Autodesk Inventor part; units mm, degrees
ref_plane "YZ Plane" through (0, 0, 0) normal (1, 0, 0) x (0, 1, 0)
ref_plane "XZ Plane" through (0, 0, 0) normal (0, 1, 0) x (-1, 0, 0)
ref_plane "XY Plane" through (0, 0, 0) normal (0, 0, 1) x (1, 0, 0)
sketch "Sketch1" plane through (0, 0, 0) normal (0, 0, 1) x (1, 0, 0)
  line L0 (0, 0) -> (25.4, 0)
  line L1 (25.4, 0) -> (25.4, -50.8)
  line L2 (25.4, -50.8) -> (0, -50.8)
  line L3 (0, -50.8) -> (0, 0)
  line L4 (22.225, -3.175) -> (3.175, -3.175)
  line L5 (3.175, -3.175) -> (3.175, -47.625)
  line L6 (3.175, -47.625) -> (22.225, -47.625)
  line L7 (22.225, -47.625) -> (22.225, -3.175)
  dimension "d0" = 25.4
  dimension "d1" = 50.8
  dimension "d2" = 3.175
  dimension "d3" = 3.175
  dimension "d4" = 3.175
  dimension "d5" = 3.175
extrude "Extrusion1" add sketch "Sketch1" along normal blind 76.2
sketch "Sketch2" plane through (0, -50.8, 0) normal (-1, 0, 0) x (0, 0, 1)
  circle A0 centre (57.15, 25.4) radius 14.2875
  line L0 (76.2, 50.8) -> (76.2, 0)
  line L1 (0, 50.8) -> (76.2, 50.8)
  dimension "d8" = 28.575
  dimension "d9" = 19.05
  dimension "d10" = 25.4
extrude "Extrusion2" cut sketch "Sketch2" against normal through all
sketch "Sketch3" plane through (0, -50.8, 0) normal (-1, 0, 0) x (0, 0, 1)
  line L0 (76.2, 47.625) -> (76.2, 3.175)
  line L1 (76.2, 31.75) -> (57.15, 50.8)
  line L2 (0, 50.8) -> (76.2, 50.8)
  line L3 (76.2, 0) -> (76.2, 50.8)
  line L4 (57.15, 50.8) -> (76.2, 50.8)
  line L5 (76.2, 50.8) -> (76.2, 31.75)
  dimension "d13" = 135
  dimension "d14" = 19.05
extrude "Extrusion3" cut sketch "Sketch3" against normal through all
sketch "Sketch4" plane through (0, -50.8, 0) normal (-1, 0, 0) x (0, 0, 1)
  circle A0 centre (12.7, 12.7) radius 3.3734
  circle A1 centre (12.7, 38.1) radius 3.3734
  line L0 (0, 50.8) -> (57.15, 50.8)
  line L1 (0, 0) -> (0, 50.8)
  dimension "d17" = 6.7469
  dimension "d18" = 12.7
  dimension "d19" = 38.1
  dimension "d20" = 12.7
  dimension "d21" = 12.7
extrude "Extrusion4" cut sketch "Sketch4" against normal blind 25.4
properties part number "flywheelsupport2" material "Aluminum 6061"
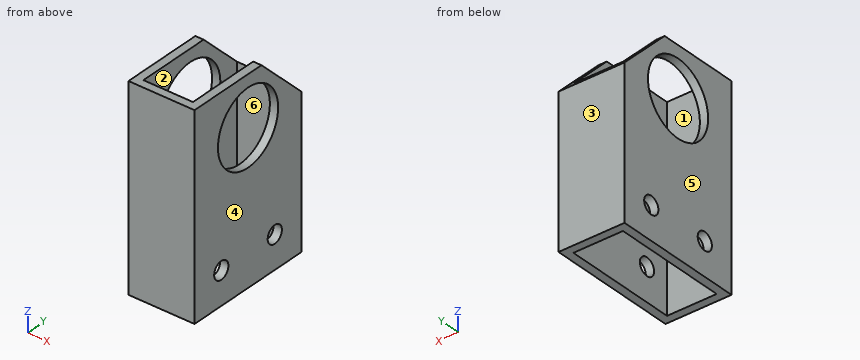
Geometry check sheet. Reference: the model listing, model coordinates, mm. Face numbers are marked on the shaded views. A direction names the side the tool comes from. Give positions to 0.01 mm unless a question says otherwise; leave off trailing zeros. Loops run counter-clockwise (first coordinate to the right, second up) from the corner with the lowest first, then second, coordinate; pieces in that order, holes last. Notation, with made-up numbers: (72.5, -13) - (115.5, -13) arc R31 ccw to (115.5, 20) - close; hole circle Ø5 at (42, 10.25). An arc over 180 degrees is marked (long way). Use CSV: the item, a comma, the result in double quotes. Start each with the question number.
Q1. Go/stop test with a flat-tipped pin: pin 1 Ø6 at (x, y) = (21, -13) entering from +Z. Record where the tip stops, or that it passes through.
Q2. Access from +Z, -Z, +X, -X, +Y, -Y to the whole of each face (thin tool, end or side, straight path). Record for the marked faces 5 and 6.
Q3. Section check C-C, the plane z = 24.5. Record the cut outline in (x, y) (3 decimals), and give its area (3 significant figures).
Q4. Section check D-D, the plane z = 12.7. Record the cut outline in (x, y) (3 decimals), and give its area (3 significant figures).
Q5. Section check A-A, the plane y = -44. Record the cut outline in (x, z) (3 decimals), and give its area (3 significant figures).
Q6. Release check for a two-part mould opening along X. For the marked faces 1, 2, 3 and 4 record: +X half, -X half, draft (parallel to the pull), parting line (faces both ways), or undercut.
Q7. Scan lines: probe 1 along Y at (x, z) = (1.4, 12.7); probe 2 along X at (y, z) = (-44, 25) (3 decimals); probe 3 along Y at (x, z) = (3.5, 24.5) (3 decimals). Record each from-to range of solid material in increasing order. Write a range as from..to.
Q8. Section check B-B, the plane x = 13.75. Record the cut outline in (y, z) (3 decimals).
Findings below:
1,pin 1,"stops at z = 72.89"
2,face 5,"+Z, -Z, -X, +Y, -Y"
2,face 6,"+Z, -Z"
3,outline,"(0, -50.8) - (25.4, -50.8) - (25.4, 0) - (0, 0) - close; hole (3.175, -47.625) - (22.225, -47.625) - (22.225, -3.175) - (3.175, -3.175) - close"
3,area,"444 mm^2"
4,outline,"(0, -50.8) - (25.4, -50.8) - (25.4, -41.473) - (22.225, -41.473) - (22.225, -47.625) - (3.175, -47.625) - (3.175, -41.473) - (0, -41.473) - close; (0, -34.727) - (3.175, -34.727) - (3.175, -16.073) - (0, -16.073) - close; (0, -9.327) - (3.175, -9.327) - (3.175, -3.175) - (22.225, -3.175) - (22.225, -9.327) - (25.4, -9.327) - (25.4, 0) - (0, 0) - close; (22.225, -34.727) - (25.4, -34.727) - (25.4, -16.073) - (22.225, -16.073) - close"
4,area,"358 mm^2"
5,outline,"(0, 0) - (3.175, 0) - (3.175, 76.2) - (0, 76.2) - close; (22.225, 0) - (25.4, 0) - (25.4, 76.2) - (22.225, 76.2) - close"
5,area,"484 mm^2"
6,face 1,"undercut"
6,face 2,"undercut"
6,face 3,"draft"
6,face 4,"+X half"
7,probe 1,"y = -50.8..-41.47, -34.73..-16.07, -9.33..0"
7,probe 2,"x = 0..3.175, 22.225..25.4"
7,probe 3,"y = -50.8..-47.625, -3.175..0"
8,outline,"(-50.8, 0) - (-47.625, 0) - (-47.625, 76.2) - (-50.8, 76.2) - close; (-3.175, 0) - (0, 0) - (0, 57.15) - (-3.175, 60.325) - close"
